```python
from build123d import *

# Parameters (mm, degrees)
F0_W      = 50
F0_H      = 10
F1_DEPTH  = 45
F2_R      = 2.5781
F3_DEPTH  = 25
F4_R      = 7.5
F5_DEPTH  = 10.001
F6_R      = 2.5
F7_DEPTH  = 25
F8_W      = 20
F8_H      = 15.5
F9_DEPTH  = 25
F8_R      = 2.5
F8_R_2    = 2.5781
F8_W_2    = 25
F8_H_2    = 4
F10_DEPTH = 8
F11_R     = 3
F12_R     = 2


# Not quite as in the source:
# - a feature of the source that left no trace in its solid (it failed there, or was rolled back) is left out


with BuildPart() as f1:
    # F0 (on Top) → F1 (new body)
    with BuildSketch(Plane.XY):
        Rectangle(F0_W, F0_H)
    extrude(amount=F1_DEPTH)

    # F2 (on face) → F3 (cut)
    with BuildSketch(Plane.XZ.offset(5)):
        with Locations((13, 37.5)):
            Circle(F2_R)
        with Locations((13, 7.5)):
            Circle(F2_R)
    extrude(amount=-F3_DEPTH, mode=Mode.SUBTRACT)

    # F4 (on face) → F5 (cut, through all)
    with BuildSketch(Plane.XZ.offset(5)):
        with Locations((13, 22.5)):
            Circle(F4_R)
    extrude(amount=-F5_DEPTH, mode=Mode.SUBTRACT)

    # F6 (on face) → F7 (cut)
    with BuildSketch(Plane.XZ.offset(5)):
        with Locations((6, 5)):
            Circle(F6_R)
        with Locations((6, 40)):
            Circle(F6_R)
        with Locations((20, 5)):
            Circle(F6_R)
        with Locations((20, 40)):
            Circle(F6_R)
        with Locations((6, 12)):
            Circle(F6_R)
        with Locations((6, 33)):
            Circle(F6_R)
        with Locations((20, 12)):
            Circle(F6_R)
        with Locations((20, 33)):
            Circle(F6_R)
    extrude(amount=-F7_DEPTH, mode=Mode.SUBTRACT)

    # F8 (on face) → F9 (cut)
    with BuildSketch(Plane.XZ.offset(5)):
        with Locations((-15, 7.75)):
            Rectangle(F8_W, F8_H)
        with Locations((-15, 37.25)):
            Rectangle(F8_W, F8_H)
    extrude(amount=-F9_DEPTH, mode=Mode.SUBTRACT)

    # F8 (on face) → F10 (cut)
    with BuildSketch(Plane.XZ.offset(5)):
        with BuildLine():
            Line((-5, 29.5), (0, 29.5))
            Line((0, 29.5), (10.3074175964, 29.5))
            ThreePointArc((10.3074175964, 29.5), (17.2459175671, 28.6824092402), (20.5, 22.5))
            ThreePointArc((20.5, 22.5), (17.2459175671, 16.3175907598), (10.3074175964, 15.5))
            Line((10.3074175964, 15.5), (0, 15.5))
            Line((0, 15.5), (-5, 15.5))
            Line((-5, 15.5), (-5, 0))
            Line((-5, 0), (25, 0))
            Line((25, 0), (25, 45))
            Line((25, 45), (-5, 45))
            Line((-5, 45), (-5, 29.5))
        make_face()
        with Locations((6, 5)):
            Circle(F8_R, mode=Mode.SUBTRACT)
        with Locations((20, 5)):
            Circle(F8_R, mode=Mode.SUBTRACT)
        with Locations((13, 7.5)):
            Circle(F8_R_2, mode=Mode.SUBTRACT)
        with Locations((6, 12)):
            Circle(F8_R, mode=Mode.SUBTRACT)
        with Locations((20, 12)):
            Circle(F8_R, mode=Mode.SUBTRACT)
        with Locations((6, 33)):
            Circle(F8_R, mode=Mode.SUBTRACT)
        with Locations((20, 33)):
            Circle(F8_R, mode=Mode.SUBTRACT)
        with Locations((6, 40)):
            Circle(F8_R, mode=Mode.SUBTRACT)
        with Locations((13, 37.5)):
            Circle(F8_R_2, mode=Mode.SUBTRACT)
        with Locations((20, 40)):
            Circle(F8_R, mode=Mode.SUBTRACT)
        with Locations((-12.5, 22.5)):
            Rectangle(F8_W_2, F8_H_2)
        with BuildLine():
            Line((10.3074175964, 24.5), (5.7715838526, 24.5))
            ThreePointArc((5.7715838526, 24.5), (5.5, 22.5), (5.7715838526, 20.5))
            Line((5.7715838526, 20.5), (10.3074175964, 20.5))
            Line((10.3074175964, 20.5), (10.3074175964, 24.5))
        make_face()
        with BuildLine():
            Line((5.7715838526, 20.5), (0, 20.5))
            Line((0, 20.5), (0, 15.5))
            Line((0, 15.5), (10.3074175964, 15.5))
            ThreePointArc((10.3074175964, 15.5), (7.4451324892, 17.4608089004), (5.7715838526, 20.5))
        make_face()
        with BuildLine():
            Line((5.7715838526, 24.5), (0, 24.5))
            Line((0, 24.5), (0, 20.5))
            Line((0, 20.5), (5.7715838526, 20.5))
            ThreePointArc((5.7715838526, 20.5), (5.5, 22.5), (5.7715838526, 24.5))
        make_face()
        with BuildLine():
            Line((0, 29.5), (0, 24.5))
            Line((0, 24.5), (5.7715838526, 24.5))
            ThreePointArc((5.7715838526, 24.5), (7.4451324892, 27.5391910996), (10.3074175964, 29.5))
            Line((10.3074175964, 29.5), (0, 29.5))
        make_face()
    extrude(amount=-F10_DEPTH, mode=Mode.SUBTRACT)

    # F11
    f11_edges = [f1.edges().sort_by_distance(p)[0] for p in [
        (25, 4, 0),
        (25, 4, 45),
        (-5, 4, 45),
        (-5, 4, 29.5),
        (-5, 4, 0),
        (-5, 4, 15.5),
    ]]
    fillet(f11_edges, radius=F11_R)

    # F12
    f12_edges = [f1.edges().sort_by_distance(p)[0] for p in [
        (0, -1, 20.5),
        (0, -1, 24.5),
    ]]
    fillet(f12_edges, radius=F12_R)


solid = f1.part
```
Here's how the part is built. I have some questions about the finished solid (model axes, mm). A direction names the side the tool comes from. Give positions to 0.01 mm unless a question says otherwise; leave off trailing zeros. Write each loop counter-clockwise with the first axis right and the second up, starting at its lowest first coordinate (ties: lowest second). Pieces come first, ordered by that corner, then holes. Notation, with made-up numbers: (85, 3.25) -> (131, 3.25) arc R6 ccw to (131, 7.25) -> close; hole circle Ø7 at (3.5, 86.5). An arc over 180 degrees is marked (long way). Use one line per item in the form item = value.
1) On a 3-axis mill with a long thin cutter (end or side, diameter ignored), from which of +Z, -Z, +X, -X, +Y, -Y can I reach the whole of each face in a straight line? I mean faces 4 (the face through (-13, 0, 15.5)), 5 (the face through (7.34, 3.99, 35.11)), 6 (the face through (-0.57, -0.94, 19.9)), 7 (the face through (0, -1, 28)), 8 (the face through (-5, 4, 37)). Say none if no direction works.
Verdict:
face_4 = -Z, -X, -Y
face_5 = +Y, -Y
face_6 = +X, -Y
face_7 = +Z, -Z, +X, -Y
face_8 = +Z, -X, +Y, -Y
2) Suppose I cut it at A-A (y = 0). Please give me the cut outline in (x, z), and give its area (3 significant figures).
Verdict:
outline = (-25, 15.5) -> (0, 15.5) -> (0, 18.5) arc R2 ccw to (-2, 20.5) -> (-25, 20.5) -> close; (-25, 24.5) -> (-2, 24.5) arc R2 ccw to (0, 26.5) -> (0, 29.5) -> (-25, 29.5) -> close
area = 248 mm2
3) We'd pull the mould along X, two halves only. Please class faces 1 (the face through (-4.14, 4.01, 0.9)), 2 (the face through (18, 4, 38.5)), 3 (the face through (24.1, 4.01, 0.86)): +X half, -X half, draft (parallel to the pull), parting line (faces both ways), or undercut.
Verdict:
face_1 = -X half
face_2 = undercut
face_3 = +X half
4) Suppose I cut it at D-D (x = -18.5). Please give me the cut outline in (y, z).
Verdict:
outline = (-5, 15.5) -> (5, 15.5) -> (5, 29.5) -> (-5, 29.5) -> (-5, 24.5) -> (3, 24.5) -> (3, 20.5) -> (-5, 20.5) -> close
5) Suppose I cut it at C-C (z = 22.5). Please give me the cut outline in (x, y).
Verdict:
outline = (-25, 3) -> (5.5, 3) -> (5.5, 5) -> (-25, 5) -> close; (20.5, 3) -> (25, 3) -> (25, 5) -> (20.5, 5) -> close
6) If I drill on L1, parallel to Z at x = 13, y = 3.7; L2, parallel to Z at x = -15, y = -1.75; L3, parallel to Y at x = 15, z = 5.5, over which ranges is the centre line in solid material (lowest first)? Write a range as [from, to].
Verdict:
L1 = [0, 4.92], [10.08, 15], [30, 34.92], [40.08, 45]
L2 = [15.5, 20.5], [24.5, 29.5]
L3 = [3, 5]
7) I'm going to push flat-ended pins straight in: pin 1 (6 mm diameter, centred on x = 6, z = 12, fed in from +Y); pin 2 (6 mm diameter, centred on x = 6, z = 40, fed in from -Y); pin 3 (4.5 mm diameter, centred on x = 6, z = 33, fed in from -Y); pin 4 (2 mm diameter, centred on y = 3.5, z = 37.5, fed in from -X). Where does each tip first touch, or does it pass through?
Verdict:
pin_1 = 5
pin_2 = 3
pin_3 = through
pin_4 = -5
8) Suppose I cut it at B-B (x = 13). Please give me the cut outline in (y, z), and give its area (3 significant figures).
Verdict:
outline = (3, 0) -> (5, 0) -> (5, 4.92) -> (3, 4.92) -> close; (3, 10.08) -> (5, 10.08) -> (5, 15) -> (3, 15) -> close; (3, 30) -> (5, 30) -> (5, 34.92) -> (3, 34.92) -> close; (3, 40.08) -> (5, 40.08) -> (5, 45) -> (3, 45) -> close
area = 39.4 mm2
